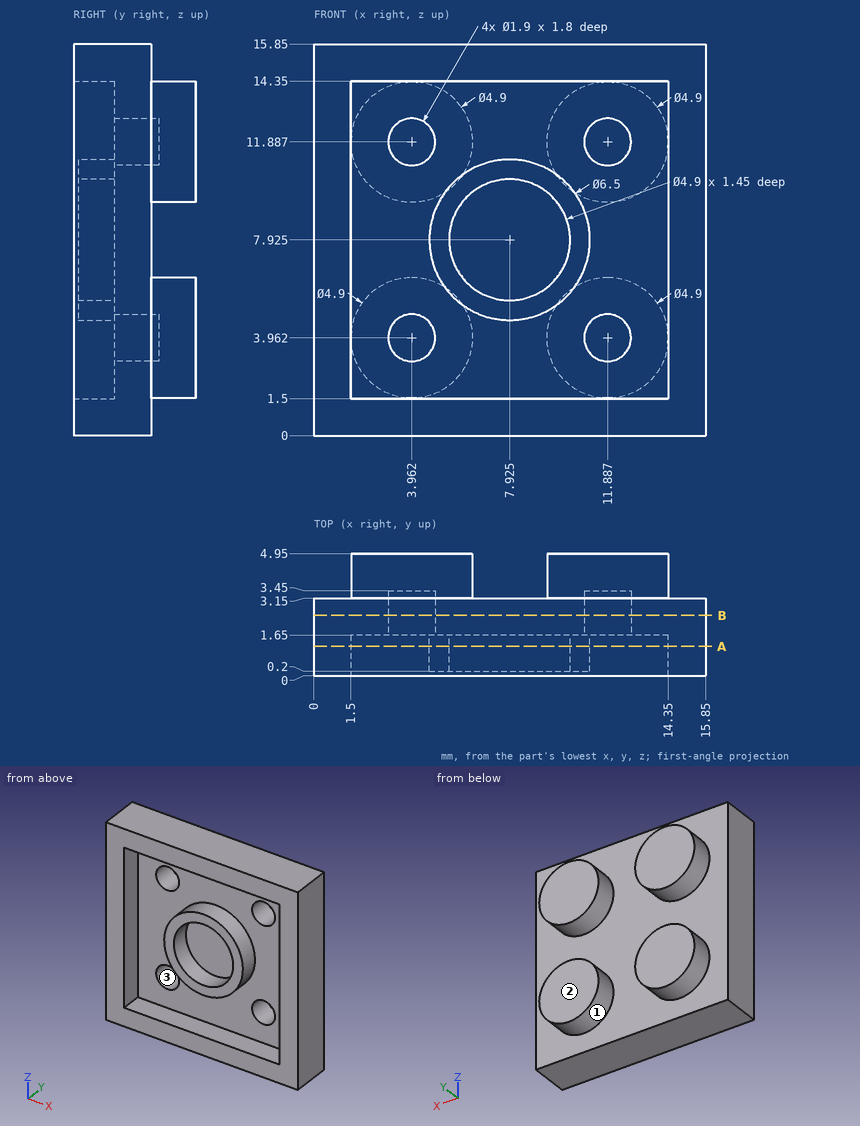
The drawing under review shows one solid part. Ordinate dimensions are in mm from its lowest x, y, z. A direction names the side the tool comes from. Give positions to 0.01 mm unless a question says otherwise; leave off trailing zeros. Loops run counter-clockwise (first coordinate to the right, second up) from the corner with the lowest first, then second, coordinate; pieces in that order, holes last. Notation, with made-up numbers: M 74,57.5 L 100,57.5 A17 cw 100,64.5 Z; hole C 87,64.25 d2. An arc over 180 degrees is marked long. Return JSON: item names as keys, results as strings. Group by question number.
Item 1: We need section B-B (y = 2.45). Give the boundary of the cut face in (x, z), and give its area (3 significant figures).
Item 2: Tool access review of the marked faces 1, 2 and 3: name each direction out of +Z, -Z, +X, -X, +Y, -Y from which nothing blocks a thin tool from reaching the whole face with its end or side.
Item 3: We need section A-A (y = 1.2). Give the number of separate pieces and of enclosed holes in the cut face.
Item 4: Insertion check: pin 1 Ø5.5 at (x, z) = (9, 8.5) entering from -Y; pin 2 Ø2 at (x, z) = (3.96, 11.89) entering from -Y; pin 3 Ø0.9 at (x, z) = (12, 12) entering from -Y. Each pin has a flat end and moves straight along its axis. Give the tip position at first contact, or say it passes through.
Item 5: For probe 1 along Z at (x, y) = (3, 0.8); probe 2 along Z at (x, y) = (8.25, 1.6); probe 3 along Z at (x, y) = (5.25, 1.4), list the stretches that pass through material, from the lowest coordinate up.
Output:
{
 "1": {"outline": "M 0,0 L 15.85,0 L 15.85,15.85 L 0,15.85 Z; hole C 3.96,3.96 d1.9; hole C 3.96,11.89 d1.9; hole C 11.89,3.96 d1.9; hole C 11.89,11.89 d1.9", "area": "240 mm^2"},
 "2": {"face 1": "+Y", "face 2": "+Z, -Z, +X, -X, +Y", "face 3": "-Y"},
 "3": {"separate pieces": "2", "enclosed holes": "2"},
 "4": {"pin 1": "stops at y = 0.2", "pin 2": "stops at y = 1.65", "pin 3": "stops at y = 3.45"},
 "5": {"probe 1": "z = 0 to 1.5, 14.35 to 15.85", "probe 2": "z = 0 to 1.5, 4.69 to 5.5, 10.35 to 11.16, 14.35 to 15.85", "probe 3": "z = 0 to 1.5, 6.08 to 9.77, 14.35 to 15.85"}
}
